Verification items for this drawing (mm, ordinates from the low corner). Coordinates: 2 decimals unless noted, no trailing zeros. Write each loop counter-clockwise with the first axis right and the second up, starting at its lowest first coordinate (ties: lowest second). Pieces come first, ordered by that corner, then holes.
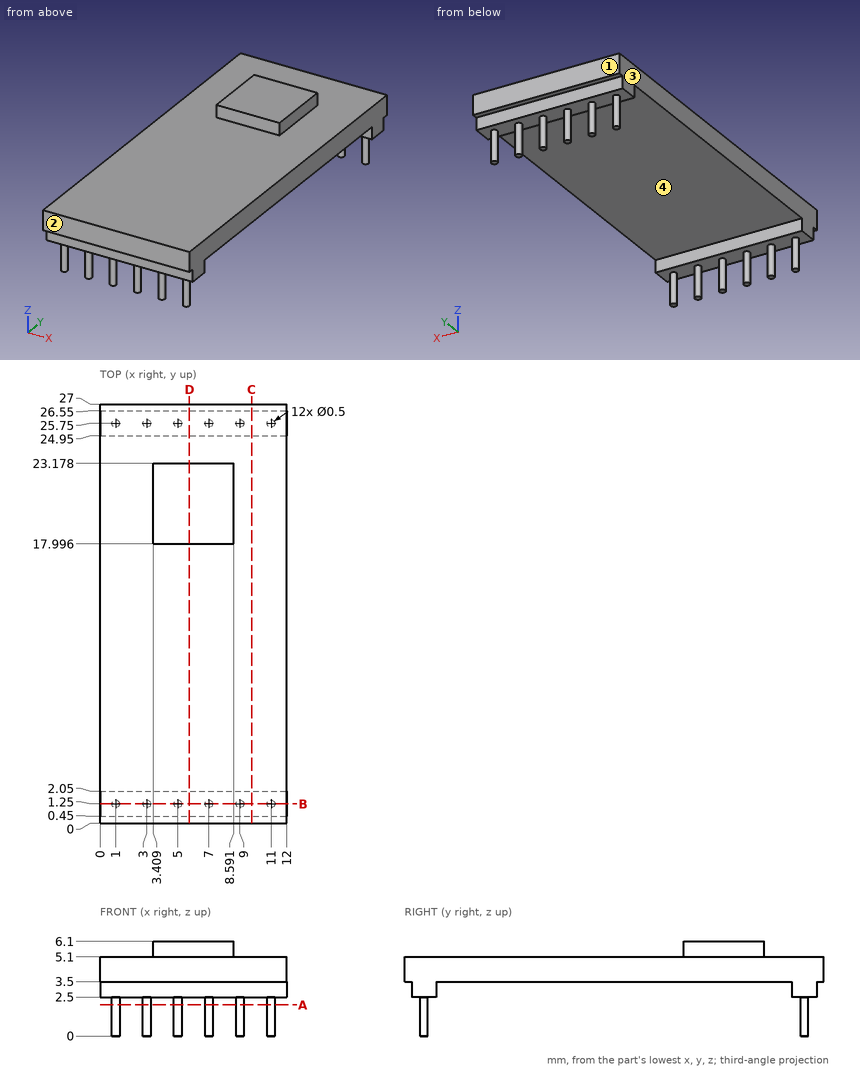
1. Sectioned sample at D-D, the plane x = 5.75. Record the boundary of the cut face in (y, z).
Computed values:
outline: (0, 3.5) - (0.45, 3.5) - (0.45, 2.5) - (2.05, 2.5) - (2.05, 3.5) - (24.95, 3.5) - (24.95, 2.5) - (26.55, 2.5) - (26.55, 3.5) - (27, 3.5) - (27, 5.1) - (23.18, 5.1) - (23.18, 6.1) - (18, 6.1) - (18, 5.1) - (0, 5.1) - close
2. Draft check along Y on the marked faces 1, 2, 3 and 4. Enter one of: released by +Y, released by -Y, zero draft, split by the parting line, or undercut.
Computed values:
face 1: released by +Y
face 2: released by -Y
face 3: zero draft
face 4: undercut
3. Sectioned sample at B-B, the plane y = 1.25. Record the boundary of the cut face in (x, z).
Computed values:
outline: (0, 2.5) - (0.75, 2.5) - (0.75, 0) - (1.25, 0) - (1.25, 2.5) - (2.75, 2.5) - (2.75, 0) - (3.25, 0) - (3.25, 2.5) - (4.75, 2.5) - (4.75, 0) - (5.25, 0) - (5.25, 2.5) - (6.75, 2.5) - (6.75, 0) - (7.25, 0) - (7.25, 2.5) - (8.75, 2.5) - (8.75, 0) - (9.25, 0) - (9.25, 2.5) - (10.75, 2.5) - (10.75, 0) - (11.25, 0) - (11.25, 2.5) - (12, 2.5) - (12, 5.1) - (0, 5.1) - close
4. Gauge pin test, flat ends, axial feed: pin 1 Ø3 at (x, y) = (6, 8.5) entering from -Z; pin 2 Ø0.5 at (y, z) = (19.5, 5.5) entering from -X; pin 3 Ø0.5 at (y, z) = (21, 5.5) entering from +X. Record the tip position at first contact, or that the pin passes through.
Computed values:
pin 1: stops at z = 3.5
pin 2: stops at x = 3.41
pin 3: stops at x = 8.59
5. Sectioned sample at A-A, the plane z = 2. Give the number of separate pieces and of enclosed holes in the cut face.
Computed values:
separate pieces: 12
enclosed holes: 0
6. Sectioned sample at C-C, the plane x = 9.75. Record the boundary of the cut face in (y, z), and give its area (3 significant figures).
Computed values:
outline: (0, 3.5) - (0.45, 3.5) - (0.45, 2.5) - (2.05, 2.5) - (2.05, 3.5) - (24.95, 3.5) - (24.95, 2.5) - (26.55, 2.5) - (26.55, 3.5) - (27, 3.5) - (27, 5.1) - (0, 5.1) - close
area: 46.4 mm2
7. Thickness scan on line 1 along Y through (x, z) = (4.25, 3); line 2 along Z through (x, y) = (10.25, 16.5); line 3 along Y through (x, z) = (5, 0.5). Record the ranges inside material, lowest first.
Computed values:
line 1: y = 0.45 to 2.05, 24.95 to 26.55
line 2: z = 3.5 to 5.1
line 3: y = 1 to 1.5, 25.5 to 26
